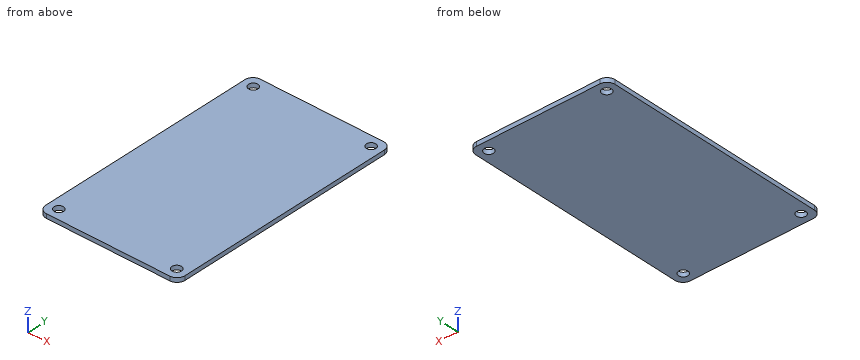
from build123d import *

# Parameters (mm, degrees)
ESQUISSE1_W                  = 52
ESQUISSE1_H                  = 89
BOSS_EXTRU_1_DEPTH           = 1.6
ENL_V_MAT_EXTRU_1_DEPTH      = 104.090057717
ENL_V_MAT_EXTRU_1_DEPTH_BACK = 104.090057717
ESQUISSE2_R                  = 1.75
CONG_1_R                     = 3


with BuildPart() as part:
    # Esquisse1 → Boss.-Extru.1 (new body)
    with BuildSketch(Plane.XY):
        with Locations((26, 44.5)):
            Rectangle(ESQUISSE1_W, ESQUISSE1_H)
    extrude(amount=BOSS_EXTRU_1_DEPTH)

    # Esquisse2 → Enlèv. mat.-Extru.1 (cut, two sides: drawn at the far end of the back side and taken through both)
    with BuildSketch(Plane.XY.offset(1.6).offset(-ENL_V_MAT_EXTRU_1_DEPTH_BACK)):
        with Locations((48, 85)):
            Circle(ESQUISSE2_R)
        with Locations(Location((48, 4, 0), (0, 0, 180))):
            Circle(ESQUISSE2_R)
        with Locations((4, 4)):
            Circle(ESQUISSE2_R)
        with Locations(Location((4, 85, 0), (0, 0, 180))):
            Circle(ESQUISSE2_R)
    extrude(amount=ENL_V_MAT_EXTRU_1_DEPTH + ENL_V_MAT_EXTRU_1_DEPTH_BACK, mode=Mode.SUBTRACT)

    # Congé1
    cong_1_edges = [part.edges().sort_by_distance(p)[0] for p in [
        (0, 89, 0.8),
        (52, 89, 0.8),
        (52, 0, 0.8),
        (0, 0, 0.8),
    ]]
    fillet(cong_1_edges, radius=CONG_1_R)


solid = part.part
For this review, take the finished solid that the model builds, in its own axes (mm). Round coordinates to 2 decimals unless told otherwise and drop trailing zeros. Loops run counter-clockwise (first coordinate to the right, second up) from the corner with the lowest first, then second, coordinate; pieces in that order, holes last. Notation, with made-up numbers: (-3, 65.5) - (24, 65.5) arc R21 cw to (24, 74.5) - close; hole circle Ø2 at (-39, 7). An arc over 180 degrees is marked (long way). Put each result on its own line as item: value. Start each with the question number.
1. Insertion check: P1, Ø5.5, axis at x = 4, y = 85, coming from the -Z side. The pin has a flat end and moves straight along its axis. Give the tip position at first contact, or say it passes through.
2. For probe 1 along Y at (x, z) = (48, 1.1); probe 2 along Y at (x, z) = (47, 0.6), list the stretches that pass through material, from the lowest coordinate up. Write a range as [from, to].
3. Consider section A-A on y = 4. State the section outline as (x, z) points, plus the area to 3 significant figures.
4. Consider section B-B on x = 4. State the section outline as (y, z) points, plus the area to 3 significant figures.
Result sheet:
1. P1: z = 0
2. probe 1: [0, 2.25], [5.75, 83.25], [86.75, 89]
2. probe 2: [0, 2.56], [5.44, 83.56], [86.44, 89]
3. outline: (0, 0) - (2.25, 0) - (2.25, 1.6) - (0, 1.6) - close; (5.75, 0) - (46.25, 0) - (46.25, 1.6) - (5.75, 1.6) - close; (49.75, 0) - (52, 0) - (52, 1.6) - (49.75, 1.6) - close
3. area: 72.0 mm^2
4. outline: (0, 0) - (2.25, 0) - (2.25, 1.6) - (0, 1.6) - close; (5.75, 0) - (83.25, 0) - (83.25, 1.6) - (5.75, 1.6) - close; (86.75, 0) - (89, 0) - (89, 1.6) - (86.75, 1.6) - close
4. area: 131 mm^2
